```python
from build123d import *

# Parameters (mm, degrees)
F0_W     = 137.16
F0_H     = 60.96
F1_DEPTH = 78.74
F2_W     = 45.72
F2_H     = 25.4
F3_DEPTH = 60.961
F4_DEPTH = 45.72
F2_W_2   = 63.5
F5_DEPTH = 15.24
F2_H_2   = 27.94
F6_DEPTH = 15.24
F7_DEPTH = 30.48


with BuildPart() as f1:
    # F0 (on Front) → F1 (new body)
    with BuildSketch(Plane.XZ):
        with Locations((45.417035, -19.691394)):
            Rectangle(F0_W, F0_H)
    extrude(amount=F1_DEPTH)

    # F2 (on face) → F3 (cut, through all)
    with BuildSketch(Plane.XY.offset(10.788606)):
        with Locations((91.137035, -66.04)):
            Rectangle(F2_W, F2_H)
    extrude(amount=-F3_DEPTH, mode=Mode.SUBTRACT)

    # F2 (on face) → F4 (cut)
    with BuildSketch(Plane.XY.offset(10.788606)):
        Polygon((86.057035, -25.4), (22.557035, -25.4), (22.557035, -53.34), (22.557035, -78.74), (68.277035, -78.74), (68.277035, -53.34), (113.997035, -53.34), (113.997035, 0), (86.057035, 0), align=None)
    extrude(amount=-F4_DEPTH, mode=Mode.SUBTRACT)

    # F2 (on face) → F5 (cut)
    with BuildSketch(Plane.XY.offset(10.788606)):
        with Locations((54.307035, -12.7)):
            Rectangle(F2_W_2, F2_H)
    extrude(amount=-F5_DEPTH, mode=Mode.SUBTRACT)

    # F2 (on face) → F6 (cut)
    with BuildSketch(Plane.XY.offset(10.788606)):
        with Locations((-0.302965, -39.37)):
            Rectangle(F2_W, F2_H_2)
    extrude(amount=-F6_DEPTH, mode=Mode.SUBTRACT)

    # F2 (on face) → F7 (cut)
    with BuildSketch(Plane.XY.offset(10.788606)):
        with Locations((-0.302965, -66.04)):
            Rectangle(F2_W, F2_H)
    extrude(amount=-F7_DEPTH, mode=Mode.SUBTRACT)


solid = f1.part
```
Can you work these out from the model? Positions are in its coordinate system, mm. A direction names the side the tool comes from. Coordinates: 2 decimals unless noted, no trailing zeros. Loops run counter-clockwise (first coordinate to the right, second up) from the corner with the lowest first, then second, coordinate; pieces in that order, holes last. Notation, with made-up numbers: (-30, 3) -> (17, 3) arc R10 cw to (17, 19) -> close; hole circle Ø1 at (59.5, -19). An arc over 180 degrees is marked (long way). Answer as a JSON object with one key per item and string values.
1) Imagine slicing it at C-C (z = -18). Please give me the cut outline in (x, y).
Results:
{"outline": "(-23.16, -53.34) -> (22.56, -53.34) -> (22.56, -25.4) -> (86.06, -25.4) -> (86.06, 0) -> (-23.16, 0) -> close"}
2) Imagine slicing it at D-D (y = -5). Please give me the cut outline in (x, z), then the cut area to 3 significant figures.
Results:
{"outline": "(-23.16, -50.17) -> (114, -50.17) -> (114, -34.93) -> (86.06, -34.93) -> (86.06, -4.45) -> (22.56, -4.45) -> (22.56, 10.79) -> (-23.16, 10.79) -> close", "area": "6,120 mm^2"}
3) Imagine slicing it at B-B (y = -37). Please give me the cut outline in (x, z).
Results:
{"outline": "(-23.16, -50.17) -> (114, -50.17) -> (114, -34.93) -> (22.56, -34.93) -> (22.56, -4.45) -> (-23.16, -4.45) -> close"}
4) For faces 1 (the face through (68.277, -66, -42)), 2 (the face through (22.557, -47, -23)), 3 (the face through (44, -39, -50.171)), 4 (the face through (-1, -53.34, -12)), 5 (the face through (54, -13, -4.451)), which set-ups out of +Z, -Z, +X, -X, +Y, -Y let a thin tool reach every point of the face, with its end or its side?
Results:
{"face 1": "+Z, -Z, +X, -Y", "face 2": "+Z, +X, -Y", "face 3": "-Z, +X, -X, +Y, -Y", "face 4": "+Z, +X, -X, -Y", "face 5": "+Z, +X, +Y, -Y"}
5) If I drill on line 1 (Y direction, x = 61, z = -14); line 2 (Z direction, x = 84, y = -10); line 3 (X direction, y = -16.5, z = -33.5), over which ranges is the centre line in solid material (lowest first)?
Results:
{"line 1": "y = -25.4 to 0", "line 2": "z = -50.17 to -4.45", "line 3": "x = -23.16 to 86.06"}
6) Imagine slicing it at A-A (x = 17). Please give me the cut outline in (y, z), then the cut area to 3 significant figures.
Results:
{"outline": "(-78.74, -50.17) -> (0, -50.17) -> (0, 10.79) -> (-25.4, 10.79) -> (-25.4, -4.45) -> (-53.34, -4.45) -> (-53.34, -19.69) -> (-78.74, -19.69) -> close", "area": "3,600 mm^2"}
7) For P1, Ø12, axis at x = 6.5, z = -8.5, coming from the -Y side; P2, Ø7.5, axis at y = -17, z = -0.5, coming from the +X side; P3, Ø8, axis at x = 60.5, z = 3, coming from the +Y side; P4, Ø1.5, axis at x = 26, z = -25.5, coming from the -Y side, each with a flat end and sliding along its axis, tell me the tip position at first contact or that it passes through.
Results:
{"P1": "stops at y = -53.34", "P2": "stops at x = 22.56", "P3": "passes through", "P4": "stops at y = -25.4"}
